Here's the drawing with two shaded views (mm, measured from the low corner). I have some questions. A direction names the side the tool comes from. Coordinates: 2 decimals unless noted, no trailing zeros. Order: outer loops, then holes, each group sorted by start corner. A loop starts at its lowest first (then second) coordinate and runs counter-clockwise, first axis right, second up. Notation, with made-up numbers: (-27.5, 81.25) -> (-19.5, 81.25) arc R19 cw to (-19.5, 85.25) -> close; hole circle Ø2 at (37, 46.25). An arc over 180 degrees is marked (long way). Answer in a Markdown table with one row per item. Add a question column.
1. Imagine slicing it at B-B on x = 3.5. Write out the boundary of the cut face in (y, z).
2. Imagine slicing it at C-C on y = 0.9. Write out the boundary of the cut face in (x, z).
3. We'd pull the mould along X, two halves only. Please class the marked faces 1, 2 and 3: pulls with the +X half, pulls with the -X half, needs draft (parallel to the pull), parting line crosses it, or undercut.
4. If I drill on line 1 along X through (y, z) = (1, 7.5); line 2 along Z through (x, y) = (3.5, 0.55); line 3 along X through (y, z) = (1.55, 7), over which ranges is the centre line in solid material (lowest first)? Write a range as [from, to].
5. Imagine slicing it at A-A on z = 7.5. Write out the boundary of the cut face in (x, y).
6. Imagine slicing it at D-D on z = 1.75. Write out the boundary of the cut face in (x, y).
7. Will these pins go through, and if not, where does the flat tip stop? pin 1 (2.5 mm diameter, centred on x = 3.5, z = 7.5, fed in from -Y); pin 2 (0.6 mm diameter, centred on y = 1, z = 0.5, fed in from -X); pin 3 (0.6 mm diameter, centred on y = 1.5, z = 10, fed in from +X).
8. On a 3-axis mill with a long thin cutter (end or side, diameter ignored), from which of +Z, -Z, +X, -X, +Y, -Y can I reach the whole of each face in a straight line? I mean the marked faces 4, 5 and 6. Say none if no direction works.
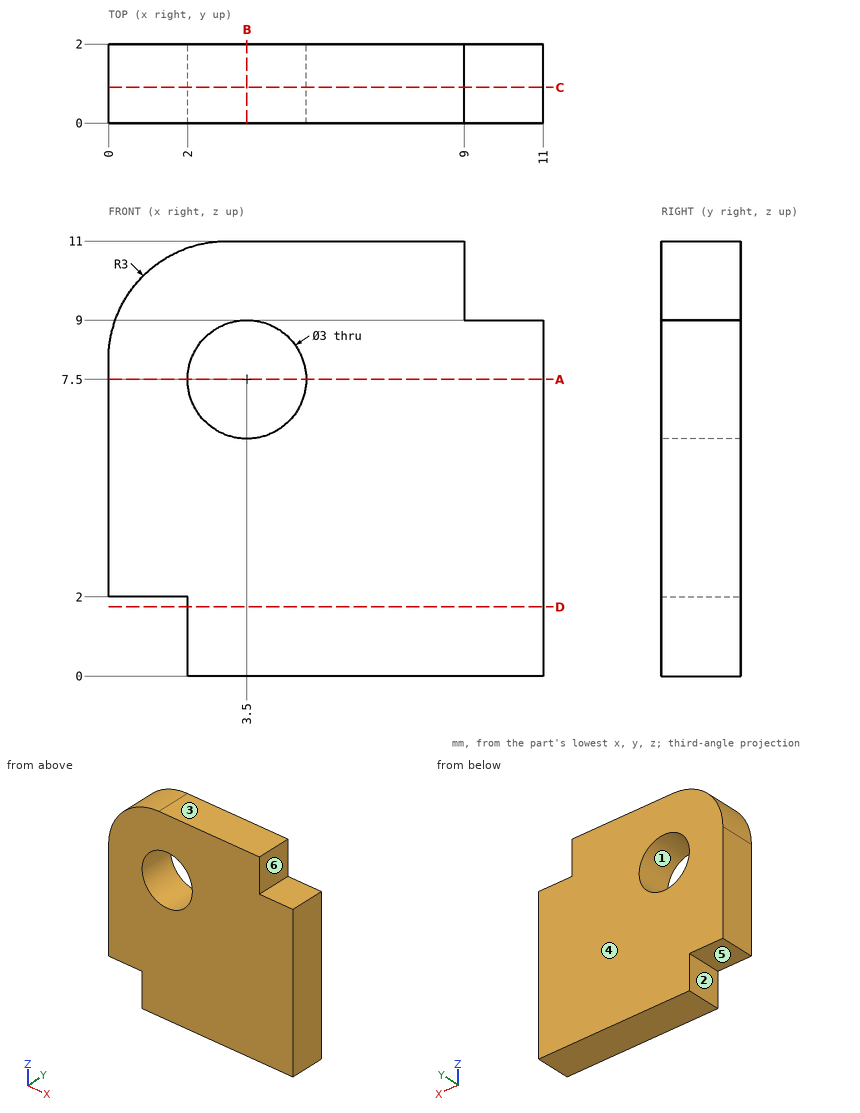
Answers follow:
| question | item | result |
|---|---|---|
| 1 | outline | (0, 0) -> (2, 0) -> (2, 6) -> (0, 6) -> close; (0, 9) -> (2, 9) -> (2, 11) -> (0, 11) -> close |
| 2 | outline | (0, 2) -> (2, 2) -> (2, 0) -> (11, 0) -> (11, 9) -> (9, 9) -> (9, 11) -> (3, 11) arc R3 ccw to (0, 8) -> close; hole circle Ø3 at (3.5, 7.5) |
| 3 | face 1 | undercut |
| 3 | face 2 | pulls with the -X half |
| 3 | face 3 | needs draft |
| 4 | line 1 | x = [0, 2], [5, 11] |
| 4 | line 2 | z = [0, 6], [9, 11] |
| 4 | line 3 | x = [0, 2.09], [4.91, 11] |
| 5 | outline | (0, 0) -> (2, 0) -> (2, 2) -> (0, 2) -> close; (5, 0) -> (11, 0) -> (11, 2) -> (5, 2) -> close |
| 6 | outline | (2, 0) -> (11, 0) -> (11, 2) -> (2, 2) -> close |
| 7 | pin 1 | passes through |
| 7 | pin 2 | stops at x = 2 |
| 7 | pin 3 | stops at x = 9 |
| 8 | face 4 | +Z, -Z, +X, -X, +Y |
| 8 | face 5 | -Z, -X, +Y, -Y |
| 8 | face 6 | +Z, +X, +Y, -Y |
